from build123d import *

# Parameters (mm, degrees)
SKETCH1_W           = 680
SKETCH1_H           = 535
SKETCH1_R           = 25
SKETCH1_R_2         = 12.5
BOSS_EXTRUDE1_DEPTH = 10


with BuildPart() as part:
    # Sketch1 → Boss-Extrude1 (new body)
    with BuildSketch(Plane(origin=(0, 0, 0), x_dir=(1, 0, 0), z_dir=(0, 1, 0))):
        Rectangle(SKETCH1_W, SKETCH1_H)
        Circle(SKETCH1_R, mode=Mode.SUBTRACT)
        with Locations((0, 133.75)):
            Circle(SKETCH1_R_2, mode=Mode.SUBTRACT)
    extrude(amount=BOSS_EXTRUDE1_DEPTH)


solid = part.part
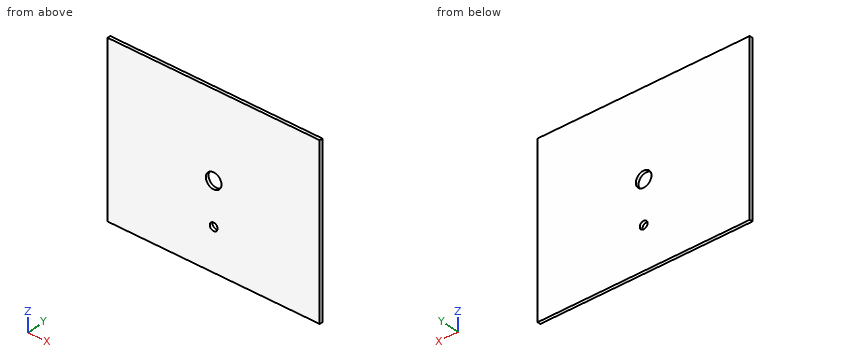
Source: CAD feature listing. Evaluate the final solid. Frame: model axes, mm. Round coordinates to 2 decimals unless told otherwise and drop trailing zeros. Order: outer loops, then holes, each group sorted by start corner. A loop starts at its lowest first (then second) coordinate and runs counter-clockwise, first axis right, second up. Notation, with made-up numbers: (74, -16.75) -> (119, -16.75) arc R14 ccw to (119, -8.75) -> close; hole circle Ø2 at (20.25, 86.5). An arc over 180 degrees is marked (long way). Answer as CSV lines item,"result".
Item 1: Section A-A, the plane x = 0. Return loops of the section in (y, z), plus the area to 3 significant figures.
A:
outline,"(0, -267.5) -> (10, -267.5) -> (10, -146.25) -> (0, -146.25) -> close; (0, -121.25) -> (10, -121.25) -> (10, -25) -> (0, -25) -> close; (0, 25) -> (10, 25) -> (10, 267.5) -> (0, 267.5) -> close"
area,"4,600 mm²"
Item 2: Pin query (flat end, axial travel): pin 1 Ø5 at (x, z) = (80, -56) entering from -Y. Return the tip coordinate at first contact, or that it passes through.
A:
pin 1,"y = 0"
Item 3: Line query: L1, parallel to Z at x = 0, y = 4.5; L2, parallel to X at y = 6.25, z = -133.75; L3, parallel to X at y = 7.75, z = 0. Output: solid intervals per line, ascending.
A:
L1,"-267.5 to -146.25, -121.25 to -25, 25 to 267.5"
L2,"-340 to -12.5, 12.5 to 340"
L3,"-340 to -25, 25 to 340"
Item 4: Section B-B, the plane z = -133.75. Return loops of the section in (x, y).
A:
outline,"(-340, 0) -> (-12.5, 0) -> (-12.5, 10) -> (-340, 10) -> close; (12.5, 0) -> (340, 0) -> (340, 10) -> (12.5, 10) -> close"
Item 5: Section C-C, the plane z = 7. Return loops of the section in (x, y).
A:
outline,"(-340, 0) -> (-24, 0) -> (-24, 10) -> (-340, 10) -> close; (24, 0) -> (340, 0) -> (340, 10) -> (24, 10) -> close"
